Verification items for the finished model (mm, model axes). Coordinates: 2 decimals unless noted, no trailing zeros. Write each loop counter-clockwise with the first axis right and the second up, starting at its lowest first coordinate (ties: lowest second). Pieces come first, ordered by that corner, then holes. Notation, with made-up numbers: (30.25, 9.5) -> (42.25, 9.5) arc R18 ccw to (42.25, 26.5) -> close; hole circle Ø1 at (24, -3). An arc over 180 degrees is marked (long way). Answer in a Markdown table with one row per item.
```python
from build123d import *

# Parameters (mm, degrees)
F0_W     = 98.442565
F0_H     = 72.012099
F0_R     = 15.107645
F1_DEPTH = 30.8957
F2_R     = 5.08
F3_SIZE  = 5.08


with BuildPart() as f1:
    # F0 (on Front) → F1 (new body)
    with BuildSketch(Plane.XZ):
        with Locations((-16.359476, 6.18827)):
            Rectangle(F0_W, F0_H)
        with Locations((-27.442385, 9.414453)):
            Circle(F0_R, mode=Mode.SUBTRACT)
    extrude(amount=F1_DEPTH)

    # F2
    f2_edges = [f1.edges().sort_by_distance(p)[0] for p in [
        (-16.359476, -30.8957, -29.817779),
    ]]
    fillet(f2_edges, radius=F2_R)

    # F3
    f3_edges = [f1.edges().sort_by_distance(p)[0] for p in [
        (-16.359476, -30.8957, 42.19432),
    ]]
    chamfer(f3_edges, length=F3_SIZE)


solid = f1.part
```
1. Sectioned sample at A-A, the plane x = -36. Record the cut outline in (y, z), and give its area (3 significant figures).
Findings below:
| item | result |
|---|---|
| outline | (-30.9, -24.74) arc R5.08 ccw to (-25.82, -29.82) -> (0, -29.82) -> (0, -3.04) -> (-30.9, -3.04) -> close; (-30.9, 21.86) -> (0, 21.86) -> (0, 42.19) -> (-25.82, 42.19) -> (-30.9, 37.11) -> close |
| area | 1,440 mm² |
2. Release check for a two-part mould opening along X. For faces 1 (the face through (-13.5, -15.2, 3.6)), 2 (the face through (32.862, -15, 6)), 3 (the face through (-65.581, -15, 6)), 4 (the face through (-6, -30.896, 7)) record: released by +X, released by -X, zero draft, split by the parting line, or undercut.
Findings below:
| item | result |
|---|---|
| face 1 | undercut |
| face 2 | released by +X |
| face 3 | released by -X |
| face 4 | zero draft |
3. Sectioned sample at D-D, the plane y = -28. Record the cut outline in (x, z).
Findings below:
| item | result |
|---|---|
| outline | (-65.58, -29.32) -> (32.86, -29.32) -> (32.86, 40.01) -> (-65.58, 40.01) -> close; hole circle Ø30.22 at (-27.44, 9.41) |
4. Material ranges on probe 1 along X at (y, z) = (-20, 9.5); probe 2 along Z at (x, y) = (-20.5, -23); probe 3 along Z at (x, y) = (-40, -4.5), recorded low to high. Write a range as from..to.
Findings below:
| item | result |
|---|---|
| probe 1 | x = -65.58..-42.55, -12.33..32.86 |
| probe 2 | z = -29.82..-4, 22.83..42.19 |
| probe 3 | z = -29.82..1.02, 17.81..42.19 |
5. Sectioned sample at B-B, the plane z = 14.5. Record the cut outline in (x, y).
Findings below:
| item | result |
|---|---|
| outline | (-65.58, -30.9) -> (-41.67, -30.9) -> (-41.67, 0) -> (-65.58, 0) -> close; (-13.22, -30.9) -> (32.86, -30.9) -> (32.86, 0) -> (-13.22, 0) -> close |
6. Sectioned sample at C-C, the plane y = -3. Record the cut outline in (x, z), and give its area (3 significant figures).
Findings below:
| item | result |
|---|---|
| outline | (-65.58, -29.82) -> (32.86, -29.82) -> (32.86, 42.19) -> (-65.58, 42.19) -> close; hole circle Ø30.22 at (-27.44, 9.41) |
| area | 6,370 mm² |
